Here's the drawing with two shaded views (mm, measured from the low corner). I have some questions. Coordinates: 2 decimals unless noted, no trailing zeros. Order: outer loops, then holes, each group sorted by start corner. A loop starts at its lowest first (then second) coordinate and runs counter-clockwise, first axis right, second up. Notation, with made-up numbers: M 88.5,22 L 126.5,22 A29 ccw 126.5,44 Z; hole C -7,-32 d11. An arc over 180 degrees is marked long. Put each result on its own line as item: value. Start each with the question number.
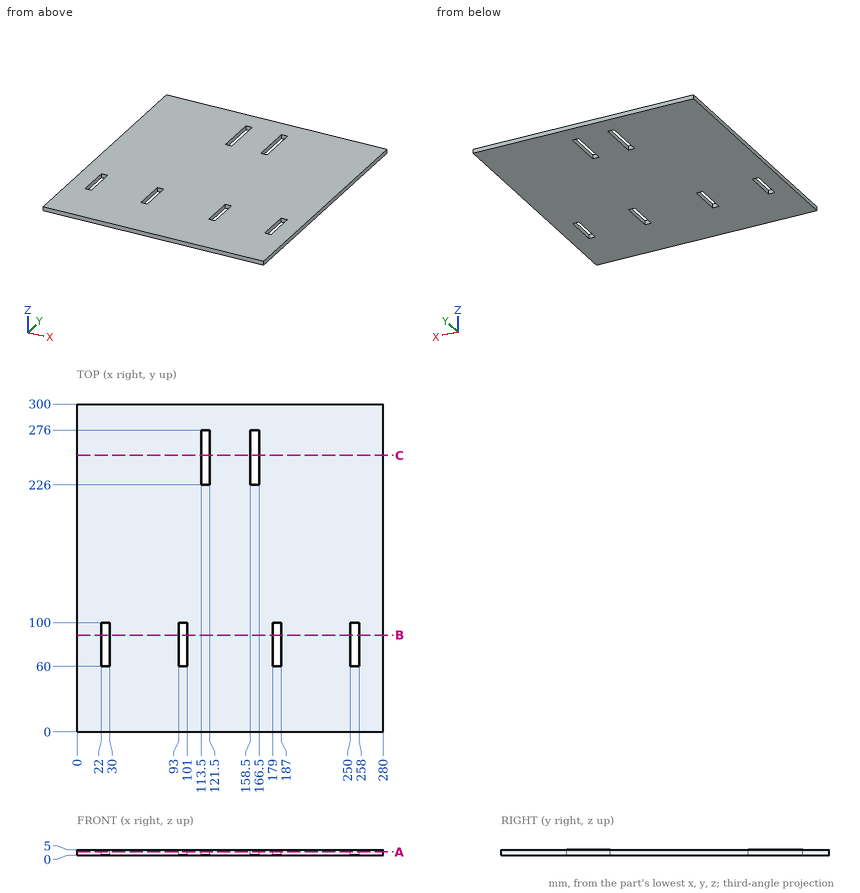
Item 1: If we section it at A-A on z = 3.3: Write out the boundary of the cut face in (x, y).
Item 2: For pin 1 Ø1.5 at (x, z) = (115.5, 3) entering from -Y, with a flat end and sliding along its axis, tell me the tip position at first contact or that it passes through.
Item 3: If we section it at B-B on y = 88.5: Write out the boundary of the cut face in (x, z).
Item 4: If we section it at C-C on y = 253: Write out the boundary of the cut face in (x, z), then the cut area to 3 significant figures.
Item 5: I need wall thicknesses on probe 1 along X at (y, z) = (92.5, 2.85); probe 2 along X at (y, z) = (262, 1.9); probe 3 along Y at (x, z) = (257, 0.4). Which ranges of each line are inside material? Lowest first, please.
Geometry check:
1. outline: M 0,0 L 280,0 L 280,300 L 0,300 Z; hole M 22,60 L 30,60 L 30,100 L 22,100 Z; hole M 93,60 L 101,60 L 101,100 L 93,100 Z; hole M 113.5,226 L 121.5,226 L 121.5,276 L 113.5,276 Z; hole M 158.5,226 L 166.5,226 L 166.5,276 L 158.5,276 Z; hole M 179,60 L 187,60 L 187,100 L 179,100 Z; hole M 250,60 L 258,60 L 258,100 L 250,100 Z
2. pin 1: stops at y = 0
3. outline: M 0,0 L 22,0 L 22,5 L 0,5 Z; M 30,0 L 93,0 L 93,5 L 30,5 Z; M 101,0 L 179,0 L 179,5 L 101,5 Z; M 187,0 L 250,0 L 250,5 L 187,5 Z; M 258,0 L 280,0 L 280,5 L 258,5 Z
4. outline: M 0,0 L 113.5,0 L 113.5,5 L 0,5 Z; M 121.5,0 L 158.5,0 L 158.5,5 L 121.5,5 Z; M 166.5,0 L 280,0 L 280,5 L 166.5,5 Z
4. area: 1,320 mm²
5. probe 1: x = 0 to 22, 30 to 93, 101 to 179, 187 to 250, 258 to 280
5. probe 2: x = 0 to 113.5, 121.5 to 158.5, 166.5 to 280
5. probe 3: y = 0 to 60, 100 to 300
